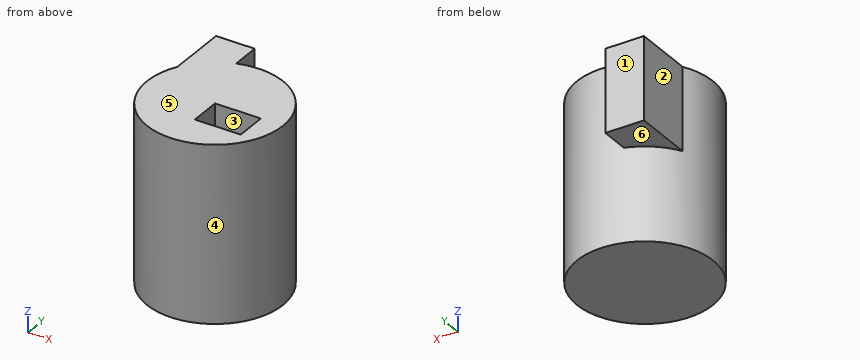
```python
from build123d import *

# Parameters (mm, degrees)
F0_R     = 55.6362832235
F1_DEPTH = 94.234
F3_R     = 55.6362832235
F3_W     = 37.5569760799
F3_H     = 25.7257614285
F4_DEPTH = 49.38980937
F6_DEPTH = 67.5356164575


with BuildPart() as f1:
    # F0 (on Top) → F1 (new body)
    with BuildSketch(Plane.XY):
        Circle(F0_R)
    extrude(amount=F1_DEPTH)

    # F3 (on face) → F4 (join)
    with BuildSketch(Plane.XY.offset(94.234)):
        Circle(F3_R)
        with Locations((18.77848804, -12.8628807142)):
            Rectangle(F3_W, F3_H, mode=Mode.SUBTRACT)
    extrude(amount=F4_DEPTH)

    # F5 (on face) → F6 (join)
    with BuildSketch(Plane.XY.offset(143.62380937)):
        with BuildLine():
            Line((-48.3959540725, 76.7373293638), (-48.3959540725, 27.4449929922))
            ThreePointArc((-48.3959540725, 27.4449929922), (-35.010462285, 43.2396061675), (-16.7768262327, 53.046527808))
            Line((-16.7768262327, 53.046527808), (-16.7768262327, 76.7373293638))
            Line((-16.7768262327, 76.7373293638), (-48.3959540725, 76.7373293638))
        make_face()
    extrude(amount=-F6_DEPTH)


solid = f1.part
```
Can you work these out from the model? Positions are in its coordinate system, mm. Face numbers are marked on the shaded views. A direction names the side the tool comes from. Give positions to 0.01 mm unless a question says otherwise; leave off trailing zeros. Write each loop counter-clockwise with the first axis right and the second up, starting at its lowest first coordinate (ties: lowest second). Pieces come first, ordered by that corner, then holes. Notation, with made-up numbers: (16.25, -7) - (68.25, -7) arc R29 ccw to (68.25, 13) - close; hole circle Ø7 at (43, 40.25). An arc over 180 degrees is marked (long way). Write item = value, one per line. Start each with the question number.
1. Thinking about a two-plate mould opening in Y: for the marked faces 1, 2, 3 and 4, which applies, released by +Y, released by -Y, zero draft, split by the parting line, or undercut?
2. On a 3-axis mill with a long thin cutter (end or side, diameter ignored), from which of +Z, -Z, +X, -X, +Y, -Y can I reach the whole of each face in a straight line? I mean the marked faces 5 and 6. Say none if no direction works.
3. For pin 1 (20.5 mm diameter, centred on y = -10.5, z = 106.5, fed in from +X); pin 2 (12 mm diameter, centred on x = -30, z = 42, fed in from -Y); pin 3 (15 mm diameter, centred on y = 53.5, z = 111.5, fed in from -X), each with a flat end and sliding along its axis, tell me the tip position at first contact or that it passes through.
4. Imagine slicing it at A-A (y = -16). Please give me the cut outline in (x, z), and give its area (3 significant figures).
5. Imagine slicing it at B-B (x = 13). Please give me the cut outline in (y, z), and give its area (3 significant figures).
6. Imagine slicing it at D-D (x = -35.5). Please give me the cut outline in (y, z), and give its area (3 significant figures).
7. Please list where these lines run through material, in increasing order: line 1 (Y direction, x = 20, z = 100); line 2 (X direction, y = -37, z = 24); line 3 (Y direction, x = -37.5, z = 109.5).
8. Imagine slicing it at C-C (z = 68.5). Please give me the cut outline in (x, y).
Worked answers:
q1.face_1 = released by +Y
q1.face_2 = zero draft
q1.face_3 = undercut
q1.face_4 = split by the parting line
q2.face_5 = +Z, +X, -X, +Y, -Y
q2.face_6 = -Z, -X, +Y
q3.pin_1 = 55.64
q3.pin_2 = -50.19
q3.pin_3 = -48.4
q4.outline = (-53.29, 0) - (53.29, 0) - (53.29, 143.62) - (37.56, 143.62) - (37.56, 94.23) - (0, 94.23) - (0, 143.62) - (-53.29, 143.62) - close
q4.area = 13,500 mm2
q5.outline = (-54.1, 0) - (54.1, 0) - (54.1, 143.62) - (0, 143.62) - (0, 94.23) - (-25.73, 94.23) - (-25.73, 143.62) - (-54.1, 143.62) - close
q5.area = 14,300 mm2
q6.outline = (-42.84, 0) - (42.84, 0) - (42.84, 76.09) - (76.74, 76.09) - (76.74, 143.62) - (-42.84, 143.62) - close
q6.area = 14,600 mm2
q7.line_1 = -51.92 to -25.73, 0 to 51.92
q7.line_2 = -41.55 to 41.55
q7.line_3 = -41.1 to 76.74
q8.outline = circle Ø111.27 at (0, 0)
